from build123d import *

# Parameters (mm, degrees)
BOSS_EXTRUDE1_DEPTH             = 9.525
CUT_EXTRUDE7_DEPTH              = 0.2
CUT_EXTRUDE8_DEPTH              = 0.2
F_29_0_136_DIAMETER_HOLE4_D     = 3.4544
F_29_0_136_DIAMETER_HOLE4_DEPTH = 13.7875
CHAMFER4_SIZE                   = 0.5


with BuildPart() as part:
    # Sketch19 → Boss-Extrude1 (new body)
    with BuildSketch(Plane(origin=(0, 4.7625, 0), x_dir=(1, 0, 0), z_dir=(0, 1, 0))):
        with BuildLine():
            Line((-14.278748413, 0.5), (-7.190320252, 0.5))
            Line((-7.190320252, 0.5), (-3.739497694, 6.477))
            Line((-3.739497694, 6.477), (3.739497694, 6.477))
            Line((3.739497694, 6.477), (7.190320252, 0.5))
            Line((7.190320252, 0.5), (14.278748413, 0.5))
            ThreePointArc((14.278748413, 0.5), (0, 14.2875), (-14.278748413, 0.5))
        make_face()
    extrude(amount=-BOSS_EXTRUDE1_DEPTH)

    # Sketch20 → Cut-Revolve1 (revolve, cut)
    with BuildSketch(Plane(origin=(0, 0, 0), x_dir=(0, -1, 0), z_dir=(-0.865794102, 0, -0.500400412))):
        Polygon((4.7625, 0), (3.7625, 0), (3.7625, -6.477), (4.7625, -7.477), align=None)
    revolve(axis=Axis((0, -4.7625, 0), (0, 1, 0)), mode=Mode.SUBTRACT)

    # Sketch21 → Cut-Revolve2 (revolve, cut)
    with BuildSketch(Plane(origin=(0, 0, 0), x_dir=(0, 1, 0), z_dir=(0.06687174, 0, 0.99776158))):
        Polygon((4.7625, -7.477), (4.7625, 0), (3.7625, 0), (3.7625, -6.477), align=None)
    revolve(axis=Axis((0, 4.7625, 0), (0, -1, 0)), mode=Mode.SUBTRACT)

    # Sketch26 → Cut-Extrude7 (cut)
    with BuildSketch(Plane(origin=(0, 4.7625, 0), x_dir=(1, 0, 0), z_dir=(0, 1, 0))):
        with BuildLine():
            Line((-14.278748413, 0.5), (-9.987492178, 0.5))
            ThreePointArc((-9.987492178, 0.5), (0, 10), (9.987492178, 0.5))
            Line((9.987492178, 0.5), (14.278748413, 0.5))
            ThreePointArc((14.278748413, 0.5), (0, 14.2875), (-14.278748413, 0.5))
        make_face()
    extrude(amount=-CUT_EXTRUDE7_DEPTH, mode=Mode.SUBTRACT)

    # Sketch27 → Cut-Extrude8 (cut)
    with BuildSketch(Plane.XZ.offset(4.7625)):
        with BuildLine():
            Line((-9.987492178, -0.5), (-14.278748413, -0.5))
            ThreePointArc((-14.278748413, -0.5), (0, -14.2875), (14.278748413, -0.5))
            Line((14.278748413, -0.5), (9.987492178, -0.5))
            ThreePointArc((9.987492178, -0.5), (0, -10), (-9.987492178, -0.5))
        make_face()
    extrude(amount=-CUT_EXTRUDE8_DEPTH, mode=Mode.SUBTRACT)

    # #29 (0.136) Diameter Hole4
    with Locations(Plane.XY.offset(-0.5)):
        with Locations((-10.368210259, 0), (10.368210259, 0)):
            Hole(F_29_0_136_DIAMETER_HOLE4_D / 2, depth=F_29_0_136_DIAMETER_HOLE4_DEPTH)

    # Chamfer4
    chamfer4_edges = [part.edges().sort_by_distance(p)[0] for p in [
        (0, 4.5625, -14.2875),
        (0, -4.5625, -14.2875),
    ]]
    chamfer(chamfer4_edges, length=CHAMFER4_SIZE)


solid = part.part
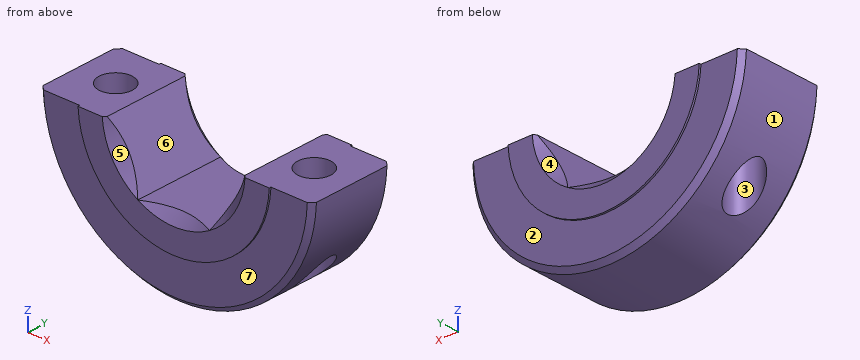
Could you check a few things on this model? Use its own coordinates, in mm. Face numbers are marked on the shaded views. A direction names the side the tool comes from. Give positions to 0.01 mm unless a question says otherwise; leave off trailing zeros. Order: outer loops, then holes, each group sorted by start corner. A loop starts at its lowest first (then second) coordinate and runs counter-clockwise, first axis right, second up.
1. Suppose I cut it at C-C (x = 0). Write out the boundary of the cut face in (y, z), plus the area to 3 significant figures.
Answers below:
outline: (-4.76, -10) - (-4.56, -10) - (-4.56, -13.79) - (-4.06, -14.29) - (4.06, -14.29) - (4.56, -13.79) - (4.56, -10) - (4.76, -10) - (4.76, -7.48) - (3.76, -6.48) - (-3.76, -6.48) - (-4.76, -7.48) - close
area: 71.4 mm2
2. Suppose I cut it at B-B (z = -2). State how many separate pieces and enclosed holes the cut face has, plus the area to 3 significant figures.
Answers below:
separate pieces: 2
enclosed holes: 2
area: 125 mm2
3. Thinking about a two-plate mould opening in X: for the marked faces 1, 2 and 3, which applies, +X half, -X half, draft (parallel to the pull), parting line (faces both ways), or undercut?
Answers below:
face 1: parting line
face 2: draft
face 3: undercut
4. Suppose I cut it at A-A (y = 0). Write out the boundary of the cut face in (x, z) (1 decimal).
Answers below:
outline: (-14.3, -0.5) arc R14.3 ccw to (-12.1, -7.6) - (-12.1, -0.5) - close; (-8.6, -11.4) arc R14.3 ccw to (8.6, -11.4) - (8.6, -0.5) - (7.2, -0.5) - (3.7, -6.5) - (-3.7, -6.5) - (-7.2, -0.5) - (-8.6, -0.5) - close; (12.1, -7.6) arc R14.3 ccw to (14.3, -0.5) - (12.1, -0.5) - close
5. For pin 1 (1 mm diameter, centred on x = -7, y = -1.5, fed in from -Z); pin 2 (3 mm diameter, centred on x = 4.5, y = 1, fed in from +Z), each with a flat end and sliding along its axis, tell me the tip position at first contact or that it passes through.
Answers below:
pin 1: stops at z = -12.72
pin 2: stops at z = -2.56
6. I need wall thicknesses on L1, parallel to X at y = 0, z = -7; L2, parallel to X at y = 0, z = -3.75; L3, parallel to X at y = 0, z = -3.5. Which ranges of each line are inside material? Lowest first, please.
Answers below:
L1: x = -12.46 to -12.1, -8.64 to 8.64, 12.1 to 12.46
L2: x = -13.79 to -12.1, -8.64 to -5.31, 5.31 to 8.64, 12.1 to 13.79
L3: x = -13.85 to -12.1, -8.64 to -5.46, 5.46 to 8.64, 12.1 to 13.85
7. Which directions (+Z, -Z, +X, -X, +Y, -Y) give clear straight access to the entire face, cutting with the end or side of a thin tool? Please do the marked faces 4, 5, 6 and 7.
Answers below:
face 4: +Z, +Y
face 5: +Z, -Y
face 6: +Z, +Y, -Y
face 7: -Z, -Y
